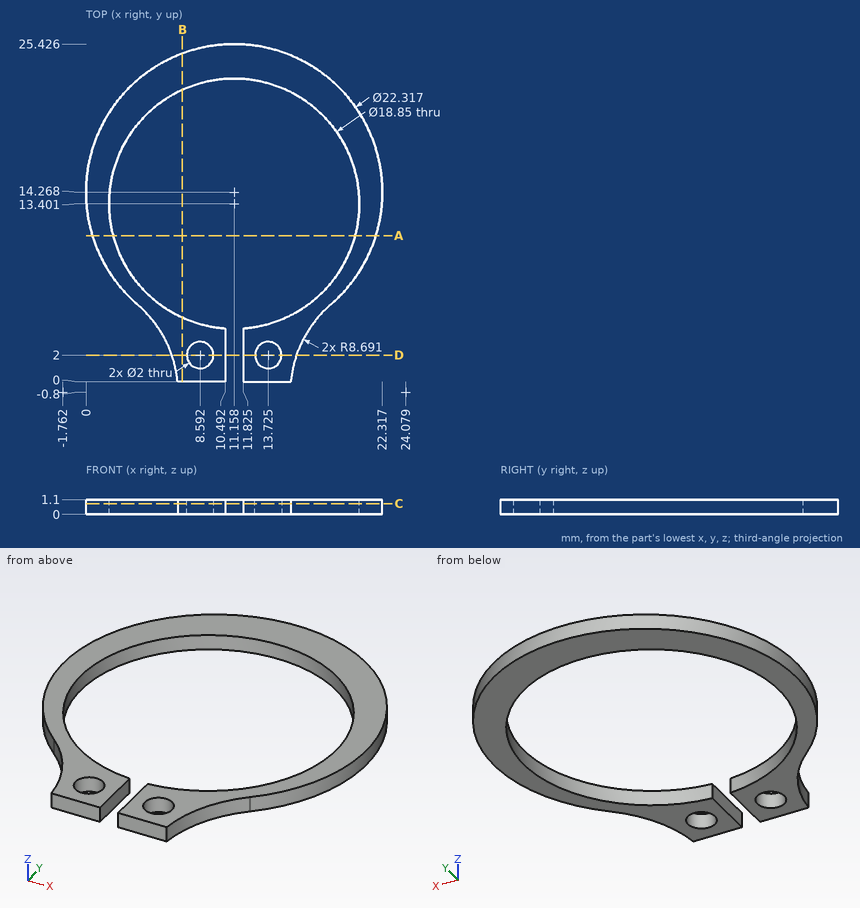
Geometry: see drawing. Coordinates: mm, zero at the bounding-box minimum. Round coordinates to 2 decimals unless told otherwise and drop trailing zeros. Order: outer loops, then holes, each group sorted by start corner. A loop starts at its lowest first (then second) coordinate and runs counter-clockwise, first axis right, second up. Notation, with made-up numbers: (52, -2) -> (72, -2) arc R38 cw to (72, 37) -> close; hole circle Ø3 at (87.5, 80.25). An arc over 180 degrees is marked (long way). Write each question's results on one line, items separated by ' | '.
Q1. Section query D-D (y = 2). Output: boundary loops of the cut face in (x, z) (1 decimal).
Response values:
outline: (6.5, 0) -> (7.6, 0) -> (7.6, 1.1) -> (6.5, 1.1) -> close; (9.6, 0) -> (10.5, 0) -> (10.5, 1.1) -> (9.6, 1.1) -> close; (11.8, 0) -> (12.7, 0) -> (12.7, 1.1) -> (11.8, 1.1) -> close; (14.7, 0) -> (15.9, 0) -> (15.9, 1.1) -> (14.7, 1.1) -> close
Q2. Section query B-B (x = 7.25). Output: boundary loops of the cut face in (y, z) (1 decimal).
Response values:
outline: (0, 0) -> (4.8, 0) -> (4.8, 1.1) -> (0, 1.1) -> close; (22, 0) -> (24.7, 0) -> (24.7, 1.1) -> (22, 1.1) -> close
Q3. Section query A-A (y = 11). Output: boundary loops of the cut face in (x, z) (1 decimal).
Response values:
outline: (0.5, 0) -> (2, 0) -> (2, 1.1) -> (0.5, 1.1) -> close; (20.3, 0) -> (21.8, 0) -> (21.8, 1.1) -> (20.3, 1.1) -> close
Q4. Ray query, line 1 along Y through (x, z) = (13.75, 0.95); line 2 along Y through (x, z) = (19, 0.55) (1 decimal); line 3 along X through (y, z) = (15.75, 1.05) (1 decimal). Return the intervals inside material, ascending.
Response values:
line 1: 0 to 1, 3 to 4.34, 22.46 to 25.12 | line 2: 6.3 to 8.2, 18.6 to 22.2 | line 3: 0.1 to 2, 20.3 to 22.2
Q5. Section query C-C (z = 0.8). Count the separate pieces of the cut face and the enclosed holes in it, and give its area (3 significant figures).
Response values:
separate pieces: 1 | enclosed holes: 2 | area: 135 mm²
Q6. Pin query (flat end, axial travel): pin 1 Ø0.6 at (y, z) = (2.5, 0.5) entering from -X; pin 2 Ø1.2 at (x, y) = (8.59, 2) entering from +Z. Return the tip coordinate at first contact, or that it passes through.
Response values:
pin 1: x = 6.15 | pin 2: through
